```python
from build123d import *

# Parameters (mm, degrees)
SKETCH_1_R      = 2.55
EXTRUDE_1_DEPTH = 1.6


with BuildPart() as part:
    # 草图1 → 凸台-拉伸1 (new body)
    with BuildSketch(Plane(origin=(0, 0, 0), x_dir=(1, 0, 0), z_dir=(0, 1, 0))):
        with BuildLine():
            Line((-738.301002862, -638.492276663), (-623.301002862, -638.492276663))
            ThreePointArc((-623.301002862, -638.492276663), (-619.765468956, -637.027810569), (-618.301002862, -633.492276663))
            ThreePointArc((-618.301002862, -633.492276663), (-619.765468956, -629.956742757), (-623.301002862, -628.492276663))
            ThreePointArc((-623.301002862, -628.492276663), (-624.715216424, -627.906490225), (-625.301002862, -626.492276663))
            Line((-625.301002862, -626.492276663), (-625.301002862, -620.922276663))
            ThreePointArc((-625.301002862, -620.922276663), (-624.715216424, -619.5080631), (-623.301002862, -618.922276663))
            ThreePointArc((-623.301002862, -618.922276663), (-619.765468956, -617.457810569), (-618.301002862, -613.922276663))
            Line((-618.301002862, -613.922276663), (-618.301002862, -543.193402957))
            ThreePointArc((-618.301002862, -543.193402957), (-619.765468956, -539.657869051), (-623.301002862, -538.193402957))
            ThreePointArc((-623.301002862, -538.193402957), (-624.715216424, -537.607616519), (-625.301002862, -536.193402957))
            Line((-625.301002862, -536.193402957), (-625.301002862, -530.623402957))
            ThreePointArc((-625.301002862, -530.623402957), (-624.715216424, -529.209189395), (-623.301002862, -528.623402957))
            ThreePointArc((-623.301002862, -528.623402957), (-619.765468956, -527.158936863), (-618.301002862, -523.623402957))
            ThreePointArc((-618.301002862, -523.623402957), (-619.765468956, -520.087869051), (-623.301002862, -518.623402957))
            Line((-623.301002862, -518.623402957), (-738.36571736, -518.55783981))
            ThreePointArc((-738.36571736, -518.55783981), (-741.901251266, -520.022305904), (-743.36571736, -523.55783981))
            Line((-743.36571736, -523.55783981), (-743.36571736, -633.55783981))
            ThreePointArc((-743.36571736, -633.55783981), (-741.855315445, -637.073994954), (-738.301002862, -638.492276663))
        make_face()
        with Locations(Location((-623.301002862, -633.492276663, 0), (0, 0, 270))):
            Circle(SKETCH_1_R, mode=Mode.SUBTRACT)
        with Locations(Location((-623.301002862, -523.623402957, 0), (0, 0, 270))):
            Circle(SKETCH_1_R, mode=Mode.SUBTRACT)
    extrude(amount=EXTRUDE_1_DEPTH)


solid = part.part
```
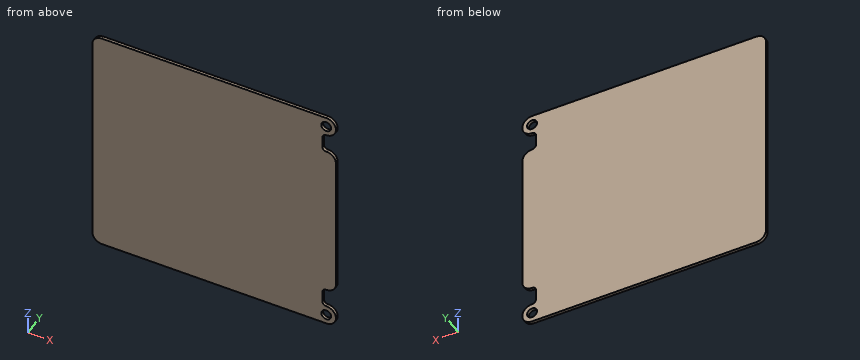
Model file for the job. Use its own axes, mm. Coordinates: 2 decimals unless noted, no trailing zeros. Write each loop counter-clockwise with the first axis right and the second up, starting at its lowest first coordinate (ties: lowest second). Pieces come first, ordered by that corner, then holes. Notation, with made-up numbers: (-4.75, -35) - (54.25, -35) arc R30 ccw to (54.25, -6) - close; hole circle Ø9 at (44.25, 58). An arc over 180 degrees is marked (long way). One line per item, written item: value. Start each with the question number.
1. Flat gauge pins, fed straight in: pin 1 (4.5 mm diameter, centred on x = -623.3, z = 523.62, fed in from -Y); pin 2 (0.5 mm diameter, centred on y = 0.5, z = 624, fed in from +X). Where does each tip first touch, or does it go through?
2. Probe line 1 (X direction, y = 1.25, z = 532.5); line 2 (Z direction, x = -717, y = 1.4); line 3 (X direction, y = 0.9, z = 614). List the from-to ranges inside material, lowest first. Write a range as from..to.
3. Slice it at A-A (z = 623.5). Write the cut outline in (x, y), plus the area to 3 significant figures.
Answers below:
1. pin 1: passes through
1. pin 2: stops at x = -625.3
2. line 1: x = -743.37..-625.3
2. line 2: z = 518.57..638.49
2. line 3: x = -743.37..-618.3
3. outline: (-743.37, 0) - (-625.3, 0) - (-625.3, 1.6) - (-743.37, 1.6) - close
3. area: 189 mm^2
